Could you check a few things on this model? Use its own coordinates, in mm. A direction names the side the tool comes from. Round coordinates to 2 decimals unless told otherwise and drop trailing zeros. Loops run counter-clockwise (first coordinate to the right, second up) from the corner with the lowest first, then second, coordinate; pieces in that order, holes last. Notation, with made-up numbers: (37.25, -30.75) -> (85.25, -30.75) arc R24 cw to (85.25, -0.75) -> close; hole circle Ø3 at (69.25, 79). An arc over 180 degrees is marked (long way). One line per item, written item: value.
```python
from build123d import *

# Parameters (mm, degrees)
F1_DEPTH = 25.4
F2_R     = 5.08
F3_R     = 5.08
F5_DEPTH = 25.4


with BuildPart() as f1:
    # F0 (on Front) → F1 (new body)
    with BuildSketch(Plane.XZ):
        Polygon((69.982089, 40.257905), (0, 0), (49.499534, -74.041769), align=None)
    extrude(amount=F1_DEPTH)

    # F2
    f2_edges = [f1.edges().sort_by_distance(p)[0] for p in [
        (34.991045, -25.4, 20.128952),
        (24.749767, -25.4, -37.020884),
        (59.740812, -25.4, -16.891932),
    ]]
    fillet(f2_edges, radius=F2_R)

    # F3
    f3_edges = [f1.edges().sort_by_distance(p)[0] for p in [
        (34.991045, 0, 20.128952),
        (24.749767, 0, -37.020884),
        (59.740812, 0, -16.891932),
    ]]
    fillet(f3_edges, radius=F3_R)

    # F4 (on face) → F5 (join)
    with BuildSketch(Plane.XZ.offset(25.4)):
        Polygon((-21.201186, 0), (7.243107, -1.693906), (33.173189, -14.002405), (35.150089, 14.359867), align=None)
    extrude(amount=F5_DEPTH)


solid = f1.part
```
Item 1: For faces 1 (the face through (41, 0, -15)), 2 (the face through (-7.178, -37.922, -0.835)), 3 (the face through (58.46, -1.53, -15.84)), 4 (the face through (34.148, -37.922, -0.02)), 5 (the face through (7.37, -37.92, 7.28)), which set-ups out of +Z, -Z, +X, -X, +Y, -Y let a thin tool reach every point of the face, with its end or its side?
Output:
face 1: +Z, -Z, +X, -X, +Y
face 2: -Z, -X, -Y
face 3: -Z, +X, +Y
face 4: -Z, +X, -Y
face 5: +Z, -X, -Y
Item 2: If we section it at B-B on x = -7.5: List the corners of the cut face in (y, z) for me.
Output:
outline: (-50.8, -0.82) -> (-25.4, -0.82) -> (-25.4, 3.49) -> (-50.8, 3.49) -> close
Item 3: Will these pins go through, and if not, where does the flat tip stop? pin 1 Ø8 at (x, z) = (3.5, 5.5) entering from +Y; pin 2 Ø1.5 at (y, z) = (-9, -24) entering from +X; pin 3 Ø1.5 at (x, z) = (48.5, 6.5) entering from -Y; pin 4 Ø4 at (x, y) = (48.5, -6.5) entering from -Z.
Output:
pin 1: stops at y = -2.08
pin 2: stops at x = 58.6
pin 3: stops at y = -25.4
pin 4: stops at z = -74.04
Item 4: If we mould it in two halves opening along Y, with no side actions, what happens to faces 6 (the face through (35.48, -12.59, 20.41)), 7 (the face through (26.366, -1.449, -36.69)), 8 (the face through (35.22, -23.87, 18.59)), 9 (the face through (19, -50.8, 0))? For each: released by +Y, released by -Y, zero draft, split by the parting line, or undercut.
Output:
face 6: zero draft
face 7: released by +Y
face 8: undercut
face 9: released by -Y
Item 5: If we section it at A-A on y = -19: List the corners of the cut face in (x, z) for me, plus the area to 3 significant figures.
Output:
outline: (0, 0) -> (49.5, -74.04) -> (69.98, 40.26) -> close
area: 3,590 mm²
Item 6: I need wall thicknesses on line 1 (Y direction, x = 52, z = -13); line 2 (Z direction, x = 8, y = -23.5); line 3 (X direction, y = -6, z = 28.5). Which ranges of each line are inside material? Lowest first, please. Write a range as from..to.
Output:
line 1: y = -25.4..0
line 2: z = -9.95..3.31
line 3: x = 49.54..67.88
Item 7: If we section it at C-C on y = -36: List the corners of the cut face in (x, z) for me, plus the area to 3 significant figures.
Output:
outline: (-21.2, 0) -> (7.24, -1.69) -> (33.17, -14) -> (35.15, 14.36) -> close
area: 632 mm²
